Geometry: final body of the model. Coordinates: model frame, mm. A direction names the side the tool comes from. Coordinates: 2 decimals unless noted, no trailing zeros. Use CSV: the item, a comma, the result in double quotes. Start each with the question number.
1. Set-up query: faces 1 (the cylindrical face through (-12.932, 4.563, 5.362)), 2 (the flat face through (0.804, 26.5, 1.6)). Return all of +Z, -Z, +X, -X, +Y, -Y with unobstructed straight access to the full face (end or side cutting, diameter ignored); none if empty.
2. Material intervals for line 1 (Y direction, x = -0.5, z = -11.25); line 2 (X direction, y = 2, z = -0.5); line 3 (Z direction, x = 6.5, y = 23.5), sorted ascending.
3. First-contact query: P1, Ø0.8, axis at x = -5, y = 26.5, coming from the -Z side; P2, Ø1.1, axis at y = 26.5, z = 1.5, coming from the +X side; P3, Ø8, axis at y = 9, z = 4.5, coming from the +X side. Flat tips, straight axial feed; report the tip coordinate or a pass-through.
4. Pull-direction query (X, two-part tool) for faces 3 (the flat face through (-5.9, 26.5, 2.304)), 4 (the flat face through (0, 0, 0)), 5 (the cylindrical face through (2.17, 18.6, 9.76)); classes: pulls with the +X half, pulls with the -X half, needs draft (parallel to the pull), parting line crosses it, or undercut.
from build123d import *

# Parameters (mm, degrees)
CHAMFER1_SIZE      = 1
FILLET1_R          = 1
FILLET2_R          = 1
CUT_EXTRUDE1_DEPTH = 1


with BuildPart() as part:
    # Sketch1 → Revolve1 (revolve)
    with BuildSketch(Plane(origin=(0, 0, 0), x_dir=(0, 1, 0), z_dir=(0, 0, 1))):
        Polygon((0, 14), (10, 14), (10, 10), (27, 10), (27, 0), (0, 0), align=None)
    revolve(axis=Axis((0, 27, 0), (0, -1, 0)))

    # Chamfer1
    chamfer1_edges = [part.edges().sort_by_distance(p)[0] for p in [
        (10, 27, 0),
    ]]
    chamfer(chamfer1_edges, length=CHAMFER1_SIZE)

    # Fillet1
    fillet1_edges = [part.edges().sort_by_distance(p)[0] for p in [
        (10, 10, 0),
    ]]
    fillet(fillet1_edges, radius=FILLET1_R)

    # Fillet2
    fillet2_edges = [part.edges().sort_by_distance(p)[0] for p in [
        (14, 10, 0),
    ]]
    fillet(fillet2_edges, radius=FILLET2_R)

    # Sketch2 → Cut-Extrude1 (cut)
    with BuildSketch(Plane(origin=(0, 27, 0), x_dir=(-1, 0, 0), z_dir=(0, 1, 0))):
        with BuildLine():
            add(Edge.make_bspline(
                [(-2.891304348, -1.376358696), (-2.893256975, -1.445784768), (-2.89704504, -1.580470179), (-2.930373434, -1.776453017), (-2.985954677, -1.958491369), (-3.06233216, -2.127831325), (-3.160586384, -2.281397406), (-3.272814945, -2.424730968), (-3.406825247, -2.550807782), (-3.555286262, -2.665606611), (-3.720516873, -2.766637543), (-3.902939881, -2.851664305), (-4.1000545, -2.925119751), (-4.312408375, -2.984347065), (-4.538102751, -3.030388297), (-4.776023597, -3.062017105), (-5.024975551, -3.08336435), (-5.19470001, -3.08574336), (-5.28125, -3.086956522)],
                knots=[0, 0, 0, 0, 1.005643061, 1.95093061, 2.870738502, 3.757832008, 4.633806625, 5.507195241, 6.389247641, 7.292512577, 8.223494331, 9.189475669, 10.205094408, 11.269007441, 12.381228937, 13.540657028, 14.745872513, 16, 16, 16, 16], degree=3))
            add(Edge.make_bspline(
                [(-5.28125, -3.086956522), (-5.360971004, -3.086063288), (-5.520031312, -3.084281097), (-5.75656703, -3.073355487), (-5.987975241, -3.055306767), (-6.21079801, -3.033603304), (-6.423346627, -3.009477077), (-6.622805279, -2.981574567), (-6.806658039, -2.949130506), (-6.923064215, -2.924650998), (-6.97826087, -2.913043478)],
                knots=[0, 0, 0, 0, 1.119729043, 2.234096861, 3.324996266, 4.379512959, 5.378439906, 6.329323539, 7.207810484, 8, 8, 8, 8], degree=3))
            Line((-6.97826087, -2.913043478), (-6.97826087, -2.130434783))
            add(Edge.make_bspline(
                [(-6.97826087, -2.130434783), (-6.919165793, -2.150682551), (-6.798419665, -2.192053842), (-6.609018112, -2.240578611), (-6.41034209, -2.286150871), (-6.20050371, -2.324223656), (-5.977458635, -2.354188802), (-5.74035588, -2.375262926), (-5.488398941, -2.389534151), (-5.315691279, -2.390703292), (-5.226902174, -2.391304348)],
                knots=[0, 0, 0, 0, 0.842364813, 1.72116351, 2.635659137, 3.591954833, 4.596841017, 5.670471508, 6.802388115, 8, 8, 8, 8], degree=3))
            add(Edge.make_bspline(
                [(-5.226902174, -2.391304348), (-5.163466632, -2.390651338), (-5.041451136, -2.389395301), (-4.865633018, -2.376263738), (-4.704182749, -2.3591435), (-4.557448129, -2.32940707), (-4.423956498, -2.295180195), (-4.303296886, -2.251625304), (-4.19565966, -2.199792452), (-4.099167106, -2.141685494), (-4.01647088, -2.074548109), (-3.943968157, -2.002194202), (-3.885784495, -1.921479924), (-3.838521468, -1.83432077), (-3.803582408, -1.740421984), (-3.779319418, -1.640031503), (-3.764056478, -1.533525867), (-3.761950623, -1.46019787), (-3.760869565, -1.422554348)],
                knots=[0, 0, 0, 0, 1.523194236, 2.929797672, 4.233142745, 5.41923506, 6.522104548, 7.540643951, 8.494207191, 9.387815665, 10.238903194, 11.04655015, 11.840679357, 12.619387111, 13.4214478, 14.239285369, 15.096122854, 16, 16, 16, 16], degree=3))
            add(Edge.make_bspline(
                [(-3.760869565, -1.422554348), (-3.762218701, -1.383440778), (-3.764854628, -1.307021088), (-3.791778823, -1.197385593), (-3.833874612, -1.095715968), (-3.895589177, -1.005041856), (-3.968114472, -0.919845819), (-4.053315168, -0.841779159), (-4.147364807, -0.766290328), (-4.290070482, -0.671359764), (-4.489755312, -0.559812554), (-4.755758112, -0.448263589), (-5.037837792, -0.336261682), (-5.327327353, -0.219443132), (-5.616743105, -0.095439779), (-5.900671358, 0.035928527), (-6.166963577, 0.186635246), (-6.367486356, 0.3361767), (-6.50758604, 0.470833926), (-6.602897854, 0.578652807), (-6.684679481, 0.696390124), (-6.760227351, 0.81988187), (-6.819332991, 0.95635363), (-6.860340608, 1.104522993), (-6.887554703, 1.264408532), (-6.890025412, 1.374880549), (-6.891304348, 1.432065217)],
                knots=[0, 0, 0, 0, 0.619815692, 1.2109895, 1.781199776, 2.357496674, 2.943929778, 3.554333405, 4.188738872, 4.856760597, 6.272963823, 7.811824644, 9.431291666, 11.092170587, 12.76691914, 14.429617761, 16.056218893, 17.616396577, 18.384212937, 19.138341755, 19.896401647, 20.65718422, 21.4332038, 22.247956952, 23.09307348, 24, 24, 24, 24], degree=3))
            add(Edge.make_bspline(
                [(-6.891304348, 1.432065217), (-6.889745465, 1.483341333), (-6.886623871, 1.586019546), (-6.860837557, 1.739445048), (-6.820282244, 1.891529982), (-6.763187009, 2.041721189), (-6.688399481, 2.186542657), (-6.59738111, 2.325382168), (-6.485582972, 2.453213148), (-6.357387336, 2.573747467), (-6.209075999, 2.684028027), (-6.042502613, 2.784628777), (-5.85495723, 2.870963409), (-5.650029948, 2.949309849), (-5.423589443, 3.011500607), (-5.17675842, 3.056055567), (-4.909488573, 3.08120208), (-4.72469023, 3.084994391), (-4.629076087, 3.086956522)],
                knots=[0, 0, 0, 0, 0.784067079, 1.570060577, 2.373452904, 3.189297991, 4.022898002, 4.862695015, 5.722463422, 6.614650011, 7.550049647, 8.544652583, 9.586108202, 10.704431291, 11.897970904, 13.172772987, 14.537200697, 16, 16, 16, 16], degree=3))
            add(Edge.make_bspline(
                [(-4.629076087, 3.086956522), (-4.575613848, 3.086610144), (-4.464505975, 3.085890284), (-4.293308173, 3.073583281), (-4.114746578, 3.058061805), (-3.933177649, 3.035827154), (-3.751912041, 3.010443569), (-3.57395579, 2.980516606), (-3.403125456, 2.948575486), (-3.292522299, 2.924611635), (-3.239130435, 2.913043478)],
                knots=[0, 0, 0, 0, 0.91416123, 1.89985515, 2.934260182, 3.979599391, 5.027947684, 6.064525625, 7.065681407, 8, 8, 8, 8], degree=3))
            Line((-3.239130435, 2.913043478), (-3.239130435, 2.217391304))
            add(Edge.make_bspline(
                [(-3.239130435, 2.217391304), (-3.357971402, 2.243749443), (-3.594474622, 2.29620429), (-3.950412242, 2.348530566), (-4.299963453, 2.385175658), (-4.530706874, 2.389285877), (-4.644021739, 2.391304348)],
                knots=[0, 0, 0, 0, 1.029411825, 2.048613503, 3.041701399, 4, 4, 4, 4], degree=3))
            add(Edge.make_bspline(
                [(-4.644021739, 2.391304348), (-4.701101178, 2.390431872), (-4.811743494, 2.388740672), (-4.971923163, 2.378342646), (-5.120237405, 2.359301917), (-5.256836907, 2.3335494), (-5.382099169, 2.301680277), (-5.495638683, 2.261191945), (-5.596829934, 2.211770598), (-5.6873755, 2.15624259), (-5.765945999, 2.093381994), (-5.835015926, 2.026647347), (-5.892681803, 1.954080686), (-5.939230398, 1.875694945), (-5.97565839, 1.792532309), (-6.003949196, 1.70494053), (-6.018307856, 1.61143275), (-6.020578052, 1.547595053), (-6.02173913, 1.514945652)],
                knots=[0, 0, 0, 0, 1.491437277, 2.890989782, 4.191431573, 5.395946596, 6.521058188, 7.565423013, 8.539223212, 9.458660202, 10.334655275, 11.163081303, 11.963306063, 12.748694206, 13.538083787, 14.331542868, 15.146677777, 16, 16, 16, 16], degree=3))
            add(Edge.make_bspline(
                [(-6.02173913, 1.514945652), (-6.020391512, 1.475835905), (-6.017758549, 1.399423684), (-5.990712947, 1.289326834), (-5.948392096, 1.187371322), (-5.889221823, 1.093867016), (-5.813847439, 1.010530917), (-5.730887666, 0.929467142), (-5.636504976, 0.853417269), (-5.494079004, 0.756044238), (-5.292632358, 0.645078177), (-5.027933357, 0.528654214), (-4.744289363, 0.419843921), (-4.455483254, 0.301879764), (-4.165028382, 0.179166441), (-3.928307462, 0.065008), (-3.744588107, -0.032987708), (-3.61583947, -0.115137783), (-3.493592228, -0.201779371), (-3.381185761, -0.297499604), (-3.27569995, -0.398738791), (-3.181404108, -0.510019231), (-3.097288568, -0.628917616), (-3.02475958, -0.756630047), (-2.962723179, -0.893416032), (-2.922268905, -1.043906372), (-2.895043236, -1.205985193), (-2.892579233, -1.318264769), (-2.891304348, -1.376358696)],
                knots=[0, 0, 0, 0, 0.667485538, 1.304126353, 1.925325377, 2.548259058, 3.18485279, 3.841928735, 4.529978862, 5.253739616, 6.789399884, 8.452896455, 10.194043647, 11.982660287, 13.786213269, 15.583473082, 16.473910229, 17.343881083, 18.192645259, 19.033319022, 19.865571682, 20.689426309, 21.522902605, 22.351690537, 23.197589349, 24.082454772, 25.007853999, 26, 26, 26, 26], degree=3))
        make_face()
        Polygon((2.39673913, -3), (1.369565217, -3), (-0.804347826, -0.057065217), (-0.804347826, -3), (-1.673913043, -3), (-1.673913043, 3), (-0.804347826, 3), (-0.804347826, 0.169836957), (1.369565217, 3), (2.336956522, 3), (-0.005434783, 0.127717391), align=None)
        Polygon((7.108695652, 2.304347826), (4.586956522, 2.304347826), (4.586956522, 0.391304348), (6.975543478, 0.391304348), (6.975543478, -0.304347826), (4.586956522, -0.304347826), (4.586956522, -3), (3.717391304, -3), (3.717391304, 3), (7.108695652, 3), align=None)
    extrude(amount=-CUT_EXTRUDE1_DEPTH, mode=Mode.SUBTRACT)


solid = part.part
Results list:
1,face 1,"+Y, -Y"
1,face 2,"+Y"
2,line 1,"y = 0 to 10"
2,line 2,"x = -13.99 to 13.99"
2,line 3,"z = -7.6 to 7.6"
3,P1,"stops at z = -8.6"
3,P2,"stops at x = 9.92"
3,P3,"stops at x = 13.99"
4,face 3,"undercut"
4,face 4,"needs draft"
4,face 5,"parting line crosses it"
